Geometry: final body of the model. Coordinates: model frame, mm. A direction names the side the tool comes from. Give positions to 0.01 mm unless a question says otherwise; leave off trailing zeros. Write each loop counter-clockwise with the first axis right and the second up, starting at its lowest first coordinate (ties: lowest second). Pieces come first, ordered by that corner, then holes.
Q1. Cut plane D-D on y = 8.75. Return the cut outline in (x, z), plus the area to 3 significant figures.
Q2. Cut plane C-C on z = 2.5. Return the cut outline in (x, y), plus the area to 3 significant figures.
Q3. Pin query (flat end, axial travel): pin 1 (4 mm diameter, centred on x = 23.5, z = 3.5, fed in from -Y); pin 2 (5 mm diameter, centred on x = -7.5, z = 12.5, fed in from -Y); pin 3 (8 mm diameter, centred on y = 18.5, z = 10.5, fed in from -X); pin 4 (1.5 mm diameter, centred on y = -3.5, z = 1.5, fed in from +X). Return the tip coordinate at first contact, or that it passes through.
Q4. Cut plane B-B on x = 25. Return the cut outline in (y, z), plus the area to 3 significant figures.
Q5. Draft query along X for faces 4 (the face through (-12.047, 20, 7)), 5 (the face through (25, 10, 3)), 6 (the face through (16, 23, 4)). Return one class per face: pulls with the +X half, pulls with the -X half, needs draft (parallel to the pull), parting line crosses it, or undercut.
Q6. Line query: L1, parallel to Y at x = 4, z = 7.7; L2, parallel to Y at x = 4, z = 3; L3, parallel to Y at x = 25, z = 4.75. Output: solid intervals per line, ascending.
Q7. Reachability of faces 1 (the face through (2, 0, 2)), 2 (the face through (6.2, 2.5, 5)), 3 (the face through (3.19, 11.34, 7.46)) from +Z, -Z, +X, -X, +Y, -Y: full face, straight path, thin tool, end or side. Return the list, or none.
Q8. Cut plane A-A on z = 8. Return the cut outline in (x, y), plus the area to 3 significant figures.
```python
from build123d import *

# Parameters (mm, degrees)
BOSS_EXTRUDE1_DEPTH = 23
SKETCH2_R           = 1.75
CUT_EXTRUDE1_DEPTH  = 10
SKETCH4_W           = 7
SKETCH4_H           = 5
BOSS_EXTRUDE2_DEPTH = 7
SKETCH6_R           = 3.75
SKETCH6_R_2         = 1.75
BOSS_EXTRUDE3_DEPTH = 5
SKETCH7_R           = 3.75
SKETCH7_R_2         = 1.75
BOSS_EXTRUDE4_DEPTH = 5
BOSS_EXTRUDE5_DEPTH = 5
BOSS_EXTRUDE6_DEPTH = 3.5
SKETCH3_R           = 1.75
CUT_EXTRUDE2_DEPTH  = 10
SKETCH12_W          = 5
SKETCH12_H          = 3
CUT_EXTRUDE3_DEPTH  = 20


with BuildPart() as part:
    # Sketch1 → Boss-Extrude1 (new body)
    with BuildSketch(Plane(origin=(0, 0, 0), x_dir=(1, 0, 0), z_dir=(0, 1, 0))):
        Polygon((18, 0), (22, 0), (35, 0), (35, -5), (35, -10), (15, -10), (15, -5), (0, -5), (0, 0), align=None)
    extrude(amount=BOSS_EXTRUDE1_DEPTH)

    # Sketch2 → Cut-Extrude1 (cut)
    with BuildSketch(Plane.XY.offset(10)):
        with Locations((4, 15)):
            Circle(SKETCH2_R)
        with Locations((25, 16)):
            Circle(SKETCH2_R)
    extrude(amount=-CUT_EXTRUDE1_DEPTH, mode=Mode.SUBTRACT)

    # Sketch4 → Boss-Extrude2 (add)
    with BuildSketch(Plane.XZ):
        with Locations((6.5, 2.5)):
            Rectangle(SKETCH4_W, SKETCH4_H)
    extrude(amount=BOSS_EXTRUDE2_DEPTH)

    # Sketch6 → Boss-Extrude3 (add)
    with BuildSketch(Plane.XY.offset(5)):
        with Locations((4, 15)):
            Circle(SKETCH6_R)
        with Locations((4, 15)):
            Circle(SKETCH6_R_2, mode=Mode.SUBTRACT)
    extrude(amount=BOSS_EXTRUDE3_DEPTH)

    # Sketch7 → Boss-Extrude4 (add)
    with BuildSketch(Plane.XY.offset(10)):
        with Locations((25, 16)):
            Circle(SKETCH7_R)
        with Locations((25, 16)):
            Circle(SKETCH7_R_2, mode=Mode.SUBTRACT)
    extrude(amount=BOSS_EXTRUDE4_DEPTH)

    # Sketch10 → Boss-Extrude5 (add)
    with BuildSketch(Plane.XY.offset(5)):
        Polygon((0, 23), (-15.047232304, 23), (-15.047232304, 15.047232304), (0, 0), align=None)
    extrude(amount=-BOSS_EXTRUDE5_DEPTH)

    # Sketch11 → Boss-Extrude6 (add)
    with BuildSketch(Plane.XY.offset(5)):
        Polygon((-12.047232304, 23), (-12.047232304, 16.289872991), (1.242640687, 3), (15, 3), (15, 6), (2.485281374, 6), (-9.047232304, 17.532513678), (-9.047232304, 23), align=None)
    extrude(amount=BOSS_EXTRUDE6_DEPTH)

    # Sketch3 → Cut-Extrude2 (cut)
    with BuildSketch(Plane.XZ):
        with Locations((25, 2.5)):
            Circle(SKETCH3_R)
    extrude(amount=-CUT_EXTRUDE2_DEPTH, mode=Mode.SUBTRACT)

    # Sketch12 → Cut-Extrude3 (cut)
    with BuildSketch(Plane.ZY.offset(-15)):
        with Locations((7.5, 1.5)):
            Rectangle(SKETCH12_W, SKETCH12_H)
    extrude(amount=-CUT_EXTRUDE3_DEPTH, mode=Mode.SUBTRACT)


solid = part.part
```
Data:
1. outline: (-8.75, 0) - (35, 0) - (35, 10) - (15, 10) - (15, 5) - (-0.26, 5) - (-0.26, 8.5) - (-4.51, 8.5) - (-4.51, 5) - (-8.75, 5) - close; hole circle Ø3.5 at (25, 2.5)
1. area: 324 mm2
2. outline: (-15.05, 15.05) - (0, 0) - (3, 0) - (3, -7) - (10, -7) - (10, 0) - (23.25, 0) - (23.25, 10) - (26.75, 10) - (26.75, 0) - (35, 0) - (35, 23) - (-15.05, 23) - close; hole circle Ø3.5 at (4, 15); hole circle Ø3.5 at (25, 16)
2. area: 1,030 mm2
3. pin 1: stops at y = 0
3. pin 2: passes through
3. pin 3: stops at x = -12.05
3. pin 4: stops at x = 10
4. outline: (0, 0) - (14.25, 0) - (14.25, 15) - (12.25, 15) - (12.25, 10) - (3, 10) - (3, 5) - (0, 5) - (0, 4.25) - (10, 4.25) - (10, 0.75) - (0, 0.75) - close; (17.75, 0) - (23, 0) - (23, 10) - (19.75, 10) - (19.75, 15) - (17.75, 15) - close
4. area: 165 mm2
5. face 4: pulls with the -X half
5. face 5: undercut
5. face 6: needs draft
6. L1: y = 3 to 6, 11.25 to 13.25, 16.75 to 18.75
6. L2: y = -7 to 13.25, 16.75 to 23
6. L3: y = 0 to 14.25, 17.75 to 23
7. face 1: +Z, -Z, -X, -Y
7. face 2: +Z, -X, -Y
7. face 3: +Z
8. outline: (-12.05, 16.29) - (1.24, 3) - (35, 3) - (35, 23) - (15, 23) - (15, 6) - (2.49, 6) - (-9.05, 17.53) - (-9.05, 23) - (-12.05, 23) - close; circle Ø7.5 at (4, 15); hole circle Ø3.5 at (4, 15); hole circle Ø3.5 at (25, 16)
8. area: 535 mm2
